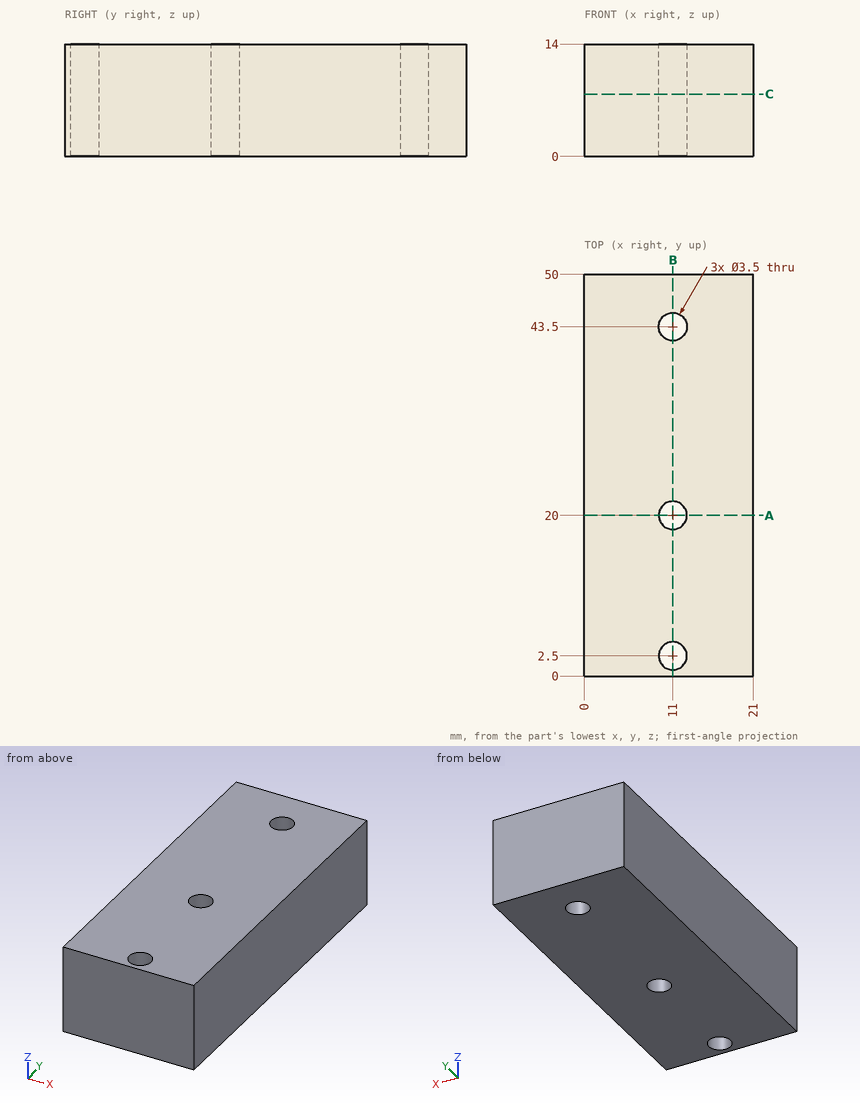
Design review of the part shown in the three views and the two pictorial views. Dimensions are in mm from the part's minimum x, y and z. Round coordinates to 2 decimals unless told otherwise and drop trailing zeros. Write each loop counter-clockwise with the first axis right and the second up, starting at its lowest first coordinate (ties: lowest second). Pieces come first, ordered by that corner, then holes. Notation, with made-up numbers: (4.25, -3) - (22.25, -3) arc R22 ccw to (22.25, 19) - close; hole circle Ø4 at (51.5, 0.25). An arc over 180 degrees is marked (long way). Write item = value, one per line. Start each with the question number.
1. Wall thickness on L1, parallel to Y at x = 11, z = 3.25; L2, parallel to Y at x = 12.5, z = 9.5; L3, parallel to X at y = 19, z = 1.5: over which ranges is each line inside the solid? List them lowest first.
2. For pin 1 Ø2 at (x, y) = (11, 43.5) entering from -Z; pin 2 Ø4 at (x, y) = (2.5, 21) entering from -Z, all flat-tipped, find the tip position at first contact; note any pin that passes through.
3. Consider section B-B on x = 11. State the section outline as (y, z) points.
4. Consider section C-C on z = 7.75. State the section outline as (x, y) points, plus the area to 3 significant figures.
5. Consider section A-A on y = 20. State the section outline as (x, z) points.
Evaluation:
q1.L1 = 0 to 0.75, 4.25 to 18.25, 21.75 to 41.75, 45.25 to 50
q1.L2 = 0 to 1.6, 3.4 to 19.1, 20.9 to 42.6, 44.4 to 50
q1.L3 = 0 to 9.56, 12.44 to 21
q2.pin_1 = through
q2.pin_2 = 0
q3.outline = (0, 0) - (0.75, 0) - (0.75, 14) - (0, 14) - close; (4.25, 0) - (18.25, 0) - (18.25, 14) - (4.25, 14) - close; (21.75, 0) - (41.75, 0) - (41.75, 14) - (21.75, 14) - close; (45.25, 0) - (50, 0) - (50, 14) - (45.25, 14) - close
q4.outline = (0, 0) - (21, 0) - (21, 50) - (0, 50) - close; hole circle Ø3.5 at (11, 2.5); hole circle Ø3.5 at (11, 20); hole circle Ø3.5 at (11, 43.5)
q4.area = 1,020 mm2
q5.outline = (0, 0) - (9.25, 0) - (9.25, 14) - (0, 14) - close; (12.75, 0) - (21, 0) - (21, 14) - (12.75, 14) - close
